Design review of the part built by this model. Coordinates are the model's own, in mm. A direction names the side the tool comes from. Give positions to 0.01 mm unless a question says otherwise; leave off trailing zeros. Order: outer loops, then holes, each group sorted by start corner. A loop starts at its lowest first (then second) coordinate and runs counter-clockwise, first axis right, second up. Notation, with made-up numbers: M 66,59.25 L 90,59.25 A10 cw 90,68.25 Z; hole C 43.5,-29.5 d4. An arc over 180 degrees is marked long. Answer as a JSON object with one key per item and string values.
from build123d import *

# Parameters (mm, degrees)
F1_DEPTH      = 6.35
F1_DEPTH_BACK = 6.35
F2_R          = 4.191
F2_R_2        = 2.5019
F3_DEPTH      = 4.064
F3_DEPTH_BACK = 24.258
F4_DEPTH      = 24.258
F5_T1_DEPTH   = 15.875
F5_T3_DEPTH   = 15.875


# Not quite as in the source:
# - a fillet or chamfer that OpenCascade refuses, or shapes differently, is made with other operations: its cross-section is extruded or revolved along the edge and cut away or added
# - a feature names something its author has since deleted; it is built from what else it names


with BuildPart() as f1:
    # F0 (on Top) → F1 (new body, two sides)
    with BuildSketch(Plane.XY) as f1_sk:
        with BuildLine():
            Line((22.098, 24.257), (17.653, 24.257))
            ThreePointArc((17.653, 24.257), (0, 6.604), (-17.653, 24.257))
            Line((-17.653, 24.257), (-22.098, 24.257))
            Line((-22.098, 24.257), (-22.098, -24.257))
            Line((-22.098, -24.257), (-14.2709804499, -24.257))
            ThreePointArc((-14.2709804498, -24.257), (-3.7215436879, -1.454770368), (16.002, -17.018))
            ThreePointArc((16.002, -17.018), (15.563229632, -20.7395436879), (14.2709804499, -24.257))
            Line((14.2709804499, -24.257), (22.098, -24.257))
            Line((22.098, -24.257), (22.098, 24.257))
        make_face()
    extrude(amount=F1_DEPTH)
    extrude(f1_sk.sketch, amount=-F1_DEPTH_BACK)

    # F2 (on Front) → F3 (cut, two sides)
    with BuildSketch(Plane.XZ) as f3_sk:
        Circle(F2_R)
        Circle(F2_R_2, mode=Mode.SUBTRACT)
        Circle(F2_R_2)
    extrude(amount=-F3_DEPTH, mode=Mode.SUBTRACT)
    extrude(f3_sk.sketch, amount=F3_DEPTH_BACK, mode=Mode.SUBTRACT)

    # F2 (on Front) → F4 (cut, through all)
    with BuildSketch(Plane.XZ):
        Circle(F2_R_2)
    extrude(amount=-F4_DEPTH, mode=Mode.SUBTRACT)

    # F5: fillet of radius 3.81 on 8 edges, made by hand

    # F5_s2 → F5_t1 (cut)
    with BuildSketch(Plane.XY):
        with BuildLine():
            add(Edge.make_bspline(
                [(-22.098, -20.447), (-22.098, -24.257), (-18.288, -24.257)],
                knots=[0, 0, 0, 1, 1, 1], degree=2, weights=[1, 1, 1]))
            Line((-18.288, -24.257), (-22.098, -24.257))
            Line((-22.098, -24.257), (-22.098, -20.447))
        make_face()
        with BuildLine():
            add(Edge.make_bspline(
                [(18.288, -24.257), (22.098, -24.257), (22.098, -20.447)],
                knots=[0, 0, 0, 1, 1, 1], degree=2, weights=[1, 1, 1]))
            Line((22.098, -20.447), (22.098, -24.257))
            Line((22.098, -24.257), (18.288, -24.257))
        make_face()
        with BuildLine():
            add(Edge.make_bspline(
                [(-18.288, 24.257), (-22.098, 24.257), (-22.098, 20.447)],
                knots=[0, 0, 0, 1, 1, 1], degree=2, weights=[1, 1, 1]))
            Line((-22.098, 20.447), (-22.098, 24.257))
            Line((-22.098, 24.257), (-18.288, 24.257))
        make_face()
        with BuildLine():
            add(Edge.make_bspline(
                [(22.098, 20.447), (22.098, 24.257), (18.288, 24.257)],
                knots=[0, 0, 0, 1, 1, 1], degree=2, weights=[1, 1, 1]))
            Line((18.288, 24.257), (22.098, 24.257))
            Line((22.098, 24.257), (22.098, 20.447))
        make_face()
    extrude(amount=F5_T1_DEPTH, mode=Mode.SUBTRACT)

    # F5_s4 → F5_t3 (cut)
    with BuildSketch(Plane.XY.offset(-15.875)):
        with BuildLine():
            add(Edge.make_bspline(
                [(-22.098, -20.447), (-22.098, -24.257), (-18.288, -24.257)],
                knots=[0, 0, 0, 1, 1, 1], degree=2, weights=[1, 1, 1]))
            Line((-18.288, -24.257), (-22.098, -24.257))
            Line((-22.098, -24.257), (-22.098, -20.447))
        make_face()
        with BuildLine():
            add(Edge.make_bspline(
                [(18.288, -24.257), (22.098, -24.257), (22.098, -20.447)],
                knots=[0, 0, 0, 1, 1, 1], degree=2, weights=[1, 1, 1]))
            Line((22.098, -20.447), (22.098, -24.257))
            Line((22.098, -24.257), (18.288, -24.257))
        make_face()
        with BuildLine():
            add(Edge.make_bspline(
                [(-18.288, 24.257), (-22.098, 24.257), (-22.098, 20.447)],
                knots=[0, 0, 0, 1, 1, 1], degree=2, weights=[1, 1, 1]))
            Line((-22.098, 20.447), (-22.098, 24.257))
            Line((-22.098, 24.257), (-18.288, 24.257))
        make_face()
        with BuildLine():
            add(Edge.make_bspline(
                [(22.098, 20.447), (22.098, 24.257), (18.288, 24.257)],
                knots=[0, 0, 0, 1, 1, 1], degree=2, weights=[1, 1, 1]))
            Line((18.288, 24.257), (22.098, 24.257))
            Line((22.098, 24.257), (22.098, 20.447))
        make_face()
    extrude(amount=F5_T3_DEPTH, mode=Mode.SUBTRACT)


solid = f1.part
(1) Draft analysis for pull direction Z (two halves, no side actions). For faces 1 (the flat face through (0, 0, 6.35)), 2 (the cylindrical face through (-4.187, 1.284, 0.184)), 3 (the flat face through (0, 0, -6.35)), state which applies: +Z half, -Z half, draft (parallel to the pull), parting line (faces both ways), or undercut.
Checked values:
{"face 1": "+Z half", "face 2": "undercut", "face 3": "-Z half"}
(2) We need section A-A (x = 0). Write out the cut boundary in (y, z).
Checked values:
{"outline": "M -1.02,-6.35 L 6.6,-6.35 L 6.6,-2.5 L 4.06,-2.5 L 4.06,-4.19 L -1.02,-4.19 Z; M -1.02,4.19 L 4.06,4.19 L 4.06,2.5 L 6.6,2.5 L 6.6,6.35 L -1.02,6.35 Z"}
(3) Tool access review of faces 4 (the flat face through (16, -24.257, 0)), 5 (the flat face through (2, 4.064, -2)): name each direction out of +Z, -Z, +X, -X, +Y, -Y from which nothing blocks a thin tool from reaching the whole face with its end or side.
Checked values:
{"face 4": "+Z, -Z, +X, -X, -Y", "face 5": "-Y"}
(4) We need section D-D (x = 17). Write out the cut boundary in (y, z), plus the area to 3 significant figures.
Checked values:
{"outline": "M -24.26,-6.35 L 19.5,-6.35 L 19.5,6.35 L -24.26,6.35 Z", "area": "556 mm^2"}
(5) We need section B-B (y = 1.5). Write out the cut boundary in (x, z), plus the area to 3 significant figures.
Checked values:
{"outline": "M -22.1,-6.35 L 22.1,-6.35 L 22.1,6.35 L -22.1,6.35 Z; hole C 0,0 d8.38", "area": "506 mm^2"}
(6) To check wall thickness, follow L1, parallel to X at y = 0.75, z = 0; L2, parallel to Z at x = 0, y = 2.1; L3, parallel to X at y = 6.2, z = 0. State the ranges of each line that lie inside material, in increasing order. Write a range as from..to.
Checked values:
{"L1": "x = -22.1..-4.19, 4.19..22.1", "L2": "z = -6.35..-4.19, 4.19..6.35", "L3": "x = -22.1..-2.5, 2.5..22.1"}
(7) We need section C-C (x = -7.5). Write out the cut boundary in (y, z).
Checked values:
{"outline": "M -2.88,-6.35 L 8.28,-6.35 L 8.28,6.35 L -2.88,6.35 Z"}
(8) Insertion check: pin 1 (2.5 mm diameter, centred on x = -1.5, z = -1.5, fed in from -Y). The pin has a flat end and moves straight along its axis. Give the tip position at first contact, or say it passes through.
Checked values:
{"pin 1": "stops at y = 4.06"}
